```python
from build123d import *

# Parameters (mm, degrees)
SKETCH2_R           = 1.5
BOSS_EXTRUDE2_DEPTH = 3
SKETCH3_W           = 27
SKETCH3_H           = 12.089495281
CUT_EXTRUDE1_DEPTH  = 10


with BuildPart() as part:
    # Sketch2 → Boss-Extrude2 (new body)
    with BuildSketch(Plane.XY):
        Polygon((143.230702788, -0.118374558), (153.230702788, -0.118374558), (157.230702788, -0.118374558), (157.230702788, 9.881625442), (153.230702788, 9.881625442), (153.230702788, 19.881625442), (156.230702788, 19.881625442), (156.230702788, 29.881625442), (153.230702788, 29.881625442), (153.230702788, 39.881625442), (156.230702788, 39.881625442), (156.230702788, 49.881625442), (153.230702788, 49.881625442), (153.230702788, 59.881625442), (157.230702788, 59.881625442), (157.230702788, 69.881625442), (153.230702788, 69.881625442), (153.230702788, 79.881625442), (157.230702788, 79.881625442), (157.230702788, 89.881625442), (153.230702788, 89.881625442), (153.230702788, 99.881625442), (156.230702788, 99.881625442), (156.230702788, 109.881625442), (153.230702788, 109.881625442), (153.230702788, 119.881625442), (156.230702788, 119.881625442), (156.230702788, 129.881625442), (153.230702788, 129.881625442), (153.230702788, 139.881625442), (157.230702788, 139.881625442), (157.230702788, 149.88750096), (153.230702788, 149.88750096), (143.230702788, 149.88750096), (143.230702788, 152.88750096), (133.230702788, 152.88750096), (133.230702788, 149.88750096), (123.230702788, 149.88750096), (123.230702788, 152.88750096), (113.230702788, 152.88750096), (113.230702788, 149.88750096), (103.230702788, 149.88750096), (103.230702788, 152.88750096), (93.230702788, 152.88750096), (93.230702788, 149.88750096), (83.230702788, 149.88750096), (83.230702788, 152.88750096), (73.230702788, 152.88750096), (73.230702788, 149.88750096), (63.230702788, 149.88750096), (63.230702788, 152.88750096), (53.230702788, 152.88750096), (53.230702788, 149.88750096), (43.230702788, 149.88750096), (43.230702788, 152.88750096), (33.230702788, 152.88750096), (33.230702788, 149.88750096), (23.230702788, 149.88750096), (23.230702788, 152.88750096), (13.230702788, 152.88750096), (13.230702788, 149.88750096), (3.230702788, 149.88750096), (-0.769297212, 149.88750096), (-0.769297212, 139.881625442), (3.230702788, 139.881625442), (3.230702788, 129.881625442), (0.230702788, 129.881625442), (0.230702788, 119.881625442), (3.230702788, 119.881625442), (3.230702788, 109.881625442), (0.230702788, 109.881625442), (0.230702788, 99.881625442), (3.230702788, 99.881625442), (3.230702788, 89.881625442), (-0.769297212, 89.881625442), (-0.769297212, 79.881625442), (3.230702788, 79.881625442), (3.230702788, 69.881625442), (-0.769297212, 69.881625442), (-0.769297212, 59.881625442), (3.230702788, 59.881625442), (3.230702788, 49.881625442), (0.230702788, 49.881625442), (0.230702788, 39.881625442), (3.230702788, 39.881625442), (3.230702788, 29.881625442), (0.230702788, 29.881625442), (0.230702788, 19.881625442), (3.230702788, 19.881625442), (3.230702788, 9.881625442), (-0.769297212, 9.881625442), (-0.769297212, -0.118374558), (3.230702788, -0.118374558), (13.230702788, -0.118374558), (13.230702788, -3.118374558), (23.230702788, -3.118374558), (23.230702788, -0.118374558), (33.230702788, -0.118374558), (33.230702788, -3.118374558), (43.230702788, -3.118374558), (43.230702788, -0.118374558), (53.230702788, -0.118374558), (53.230702788, -3.118374558), (63.230702788, -3.118374558), (63.230702788, -0.118374558), (73.230702788, -0.118374558), (73.230702788, -3.118374558), (83.230702788, -3.118374558), (83.230702788, -0.118374558), (93.230702788, -0.118374558), (93.230702788, -3.118374558), (103.230702788, -3.118374558), (103.230702788, -0.118374558), (113.230702788, -0.118374558), (113.230702788, -3.118374558), (123.230702788, -3.118374558), (123.230702788, -0.118374558), (133.230702788, -0.118374558), (133.230702788, -3.118374558), (143.230702788, -3.118374558), align=None)
        with Locations((1.730702788, 4.884563201)):
            Circle(SKETCH2_R, mode=Mode.SUBTRACT)
        with Locations((1.730702788, 64.884563201)):
            Circle(SKETCH2_R, mode=Mode.SUBTRACT)
        with Locations((154.730702788, 4.884563201)):
            Circle(SKETCH2_R, mode=Mode.SUBTRACT)
        with Locations((154.730702788, 64.884563201)):
            Circle(SKETCH2_R, mode=Mode.SUBTRACT)
        with Locations((1.730702788, 84.884563201)):
            Circle(SKETCH2_R, mode=Mode.SUBTRACT)
        with Locations((1.730702788, 144.884563201)):
            Circle(SKETCH2_R, mode=Mode.SUBTRACT)
        with Locations((154.730702788, 84.884563201)):
            Circle(SKETCH2_R, mode=Mode.SUBTRACT)
        with Locations((154.730702788, 144.884563201)):
            Circle(SKETCH2_R, mode=Mode.SUBTRACT)
    extrude(amount=BOSS_EXTRUDE2_DEPTH)

    # Sketch3 → Cut-Extrude1 (cut)
    with BuildSketch(Plane(origin=(0, 0, 0), x_dir=(-1, 0, 0), z_dir=(0, 0, -1))):
        with Locations((-127.430702788, 8.503599334)):
            Rectangle(SKETCH3_W, SKETCH3_H)
    extrude(amount=-CUT_EXTRUDE1_DEPTH, mode=Mode.SUBTRACT)


solid = part.part
```
Read the model definition and answer for the solid it produces. Units are mm, in the model's axes. Give positions to 0.01 mm unless a question says otherwise; leave off trailing zeros. Order: outer loops, then holes, each group sorted by start corner. A loop starts at its lowest first (then second) coordinate and runs counter-clockwise, first axis right, second up. Notation, with made-up numbers: (56.5, 72.25) -> (99.5, 72.25) arc R23 cw to (99.5, 81.25) -> close; hole circle Ø7 at (14, 59.5). An arc over 180 degrees is marked (long way). Write item = value, one per line.
1. Straight lines are drawn through the part: line 1 along Y through (x, z) = (135.5, 0.5); line 2 along Y through (x, z) = (124, 2.8); line 3 along X through (y, z) = (97, 1.7). For each, find the intervals that lie inside material, in ascending order.
Numbers:
line_1 = -3.12 to 2.46, 14.55 to 152.89
line_2 = -0.12 to 2.46, 14.55 to 149.89
line_3 = 3.23 to 153.23
2. A cutting plane is placed at C-C, the plane y = 32.5. Write down the section's boundary in (x, z), and give its area (3 significant figures).
Numbers:
outline = (3.23, 0) -> (153.23, 0) -> (153.23, 3) -> (3.23, 3) -> close
area = 450 mm²
3. Given pin 1 (1.5 mm diameter, centred on x = 28, z = 1, fed in from -Y); pin 2 (1.5 mm diameter, centred on y = 97, z = 2, fed in from -X); pin 3 (1.5 mm diameter, centred on y = 25, z = 1.5, fed in from -X), each flat-ended and moving along its own axis, determine where each tip first touches the part or whether it passes through.
Numbers:
pin_1 = -0.12
pin_2 = 3.23
pin_3 = 0.23
4. A cutting plane is placed at A-A, the plane z = 1.9. Count the separate pieces of the cut face and the enclosed holes in it, and give its area (3 significant figures).
Numbers:
separate_pieces = 1
enclosed_holes = 9
area = 23,100 mm²
5. A cutting plane is placed at B-B, the plane x = 69. Write down the section's boundary in (y, z), and give its area (3 significant figures).
Numbers:
outline = (-0.12, 0) -> (149.89, 0) -> (149.89, 3) -> (-0.12, 3) -> close
area = 450 mm²
